```python
from build123d import *

# Parameters (mm, degrees)
SKETCH2_W           = 37.621859492
SKETCH2_H           = 44.8
SKETCH2_R           = 11.25
SKETCH2_R_2         = 1.5
SKETCH2_R_3         = 1
SKETCH2_R_4         = 1.6
BOSS_EXTRUDE1_DEPTH = 3.5
SKETCH4_R           = 2.9
CUT_EXTRUDE1_DEPTH  = 2.5
SKETCH6_R           = 2.9
CUT_EXTRUDE2_DEPTH  = 2.5


with BuildPart() as part:
    # Sketch2 → Boss-Extrude1 (new body)
    with BuildSketch(Plane(origin=(0, 0, 0), x_dir=(1, 0, 0), z_dir=(0, 1, 0))):
        Rectangle(SKETCH2_W, SKETCH2_H)
        Circle(SKETCH2_R, mode=Mode.SUBTRACT)
        with Locations((-13, 13)):
            Circle(SKETCH2_R_2, mode=Mode.SUBTRACT)
        with Locations((13, 13)):
            Circle(SKETCH2_R_2, mode=Mode.SUBTRACT)
        with Locations((13, -13)):
            Circle(SKETCH2_R_2, mode=Mode.SUBTRACT)
        with Locations((-13, -13)):
            Circle(SKETCH2_R_2, mode=Mode.SUBTRACT)
        with Locations((8.98, 8.98)):
            Circle(SKETCH2_R_3, mode=Mode.SUBTRACT)
        with Locations((-8.98, 8.98)):
            Circle(SKETCH2_R_3, mode=Mode.SUBTRACT)
        with Locations((8.98, -8.98)):
            Circle(SKETCH2_R_3, mode=Mode.SUBTRACT)
        with Locations((-8.98, -8.98)):
            Circle(SKETCH2_R_3, mode=Mode.SUBTRACT)
        with Locations((-15.31, 18.9)):
            Circle(SKETCH2_R_4, mode=Mode.SUBTRACT)
        with Locations((15.31, 18.9)):
            Circle(SKETCH2_R_4, mode=Mode.SUBTRACT)
        with Locations((15.31, -18.9)):
            Circle(SKETCH2_R_4, mode=Mode.SUBTRACT)
        with Locations((-15.31, -18.9)):
            Circle(SKETCH2_R_4, mode=Mode.SUBTRACT)
    extrude(amount=BOSS_EXTRUDE1_DEPTH)

    # Sketch4 → Cut-Extrude1 (cut)
    with BuildSketch(Plane.XZ):
        with Locations((-13, -13)):
            Circle(SKETCH4_R)
        with Locations((13, -13)):
            Circle(SKETCH4_R)
        with Locations((13, 13)):
            Circle(SKETCH4_R)
        with Locations((-13, 13)):
            Circle(SKETCH4_R)
    extrude(amount=-CUT_EXTRUDE1_DEPTH, mode=Mode.SUBTRACT)

    # Sketch6 → Cut-Extrude2 (cut)
    with BuildSketch(Plane(origin=(0, 3.5, 0), x_dir=(1, 0, 0), z_dir=(0, 1, 0))):
        with Locations((-15.31, 18.9)):
            Circle(SKETCH6_R)
        with Locations((15.31, -18.9)):
            Circle(SKETCH6_R)
        with Locations((15.309998981, 18.900002337)):
            Circle(SKETCH6_R)
        with Locations((-15.31, -18.9)):
            Circle(SKETCH6_R)
    extrude(amount=-CUT_EXTRUDE2_DEPTH, mode=Mode.SUBTRACT)


solid = part.part
```
Work out the finished part from the listing and answer in its coordinate system (mm). A direction names the side the tool comes from. Give positions to 0.01 mm unless a question says otherwise; leave off trailing zeros. Write each loop counter-clockwise with the first axis right and the second up, starting at its lowest first coordinate (ties: lowest second). Pieces come first, ordered by that corner, then holes.
(1) Flat-ended cylindrical pins translate along their axes: pin 1 Ø3.5 at (x, z) = (15.31, 18.9) entering from +Y; pin 2 Ø3 at (x, z) = (15.31, -18.9) entering from -Y; pin 3 Ø2 at (x, z) = (13.5, 11.5) entering from -Y. Find the tip coordinate at first contact, or state that the pin passes through.
Final values:
pin 1: stops at y = 1
pin 2: passes through
pin 3: stops at y = 2.5
(2) The part is cut by section C-C on y = 1.5. Count the separate pieces of the cut face and the enclosed holes in it, plus the area to 3 significant figures.
Final values:
separate pieces: 1
enclosed holes: 13
area: 1,060 mm2
(3) Straight lines are drawn through the part: line 1 (X direction, y = 2.65, z = 18.9); line 2 (X direction, y = 2.9, z = 14); line 3 (Z direction, x = 14, y = 0.35). For each, find the intervals that lie inside material, in ascending order.
Final values:
line 1: x = -18.81 to -18.21, -12.41 to 12.41, 18.21 to 18.81
line 2: x = -18.81 to -14.12, -11.88 to 11.88, 14.12 to 18.81
line 3: z = -22.4 to -19.82, -17.98 to -15.72, -10.28 to 10.28, 15.72 to 17.98, 19.82 to 22.4
(4) The mould has two halves that part along Z. Classify faces 4 (the flat face through (12, 3.5, 0)), 5 (the flat face through (0, 2, -22.4)), 6 (the flat face through (-11.8, 2.5, -14.2)), 7 (the cylindrical face through (-9.77, 1.73, -8.37)): pulls with the +Z half, pulls with the -Z half, needs draft (parallel to the pull), parting line crosses it, or undercut.
Final values:
face 4: needs draft
face 5: pulls with the -Z half
face 6: undercut
face 7: undercut
(5) The part is cut by section D-D on x = 13. Write down the section's boundary in (y, z), plus the area to 3 significant figures.
Final values:
outline: (0, -22.4) - (3.5, -22.4) - (3.5, -20.65) - (1, -20.65) - (1, -17.15) - (3.5, -17.15) - (3.5, -14.5) - (2.5, -14.5) - (2.5, -15.9) - (0, -15.9) - close; (0, -10.1) - (2.5, -10.1) - (2.5, -11.5) - (3.5, -11.5) - (3.5, 11.5) - (2.5, 11.5) - (2.5, 10.1) - (0, 10.1) - close; (0, 15.9) - (2.5, 15.9) - (2.5, 14.5) - (3.5, 14.5) - (3.5, 17.15) - (1, 17.15) - (1, 20.65) - (3.5, 20.65) - (3.5, 22.4) - (0, 22.4) - close
area: 104 mm2
(6) The part is cut by section A-A on z = 13. Write down the section's boundary in (x, y).
Final values:
outline: (-18.81, 0) - (-15.9, 0) - (-15.9, 2.5) - (-14.5, 2.5) - (-14.5, 3.5) - (-18.81, 3.5) - close; (-11.5, 2.5) - (-10.1, 2.5) - (-10.1, 0) - (10.1, 0) - (10.1, 2.5) - (11.5, 2.5) - (11.5, 3.5) - (-11.5, 3.5) - close; (14.5, 2.5) - (15.9, 2.5) - (15.9, 0) - (18.81, 0) - (18.81, 3.5) - (14.5, 3.5) - close
(7) Which of the six approach directions +Z, -Z, +X, -X, +Y, -Y give full straight-line access (tool end or side, diameter ignored) to faces 1 (the flat face through (17, 1, 20)), 2 (the flat face through (14.2, 2.5, 11.8)), 3 (the cylindrical face through (9.934, 1.726, 8.68))?
Final values:
face 1: +Y
face 2: -Y
face 3: +Y, -Y
(8) The part is cut by section B-B on x = 0. Write down the section's boundary in (y, z).
Final values:
outline: (0, -22.4) - (3.5, -22.4) - (3.5, -11.25) - (0, -11.25) - close; (0, 11.25) - (3.5, 11.25) - (3.5, 22.4) - (0, 22.4) - close
